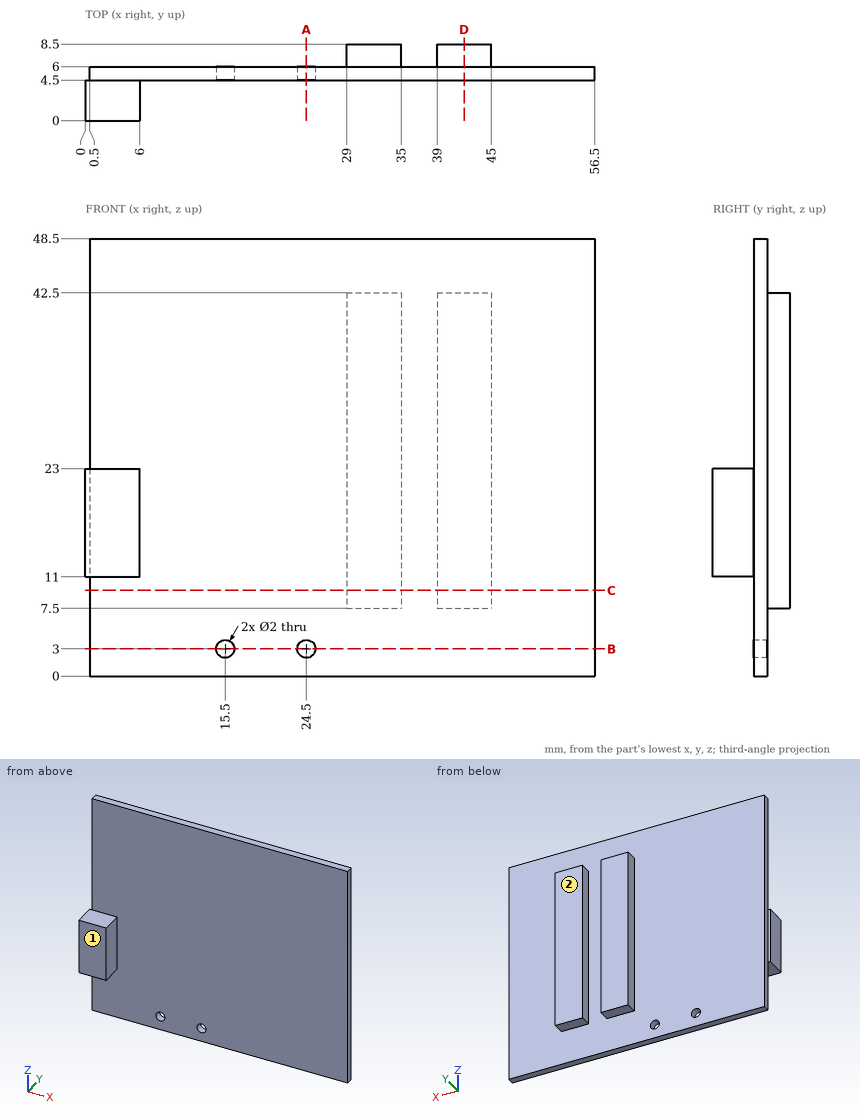
Print and shaded views of the part. All mm, measured from the part's lowest x, y and z. Coordinates: 2 decimals unless noted, no trailing zeros. Order: outer loops, then holes, each group sorted by start corner. A loop starts at its lowest first (then second) coordinate and runs counter-clockwise, first axis right, second up. Notation, with made-up numbers: M -32.75,43 L 18.25,43 A21 cw 18.25,63 Z; hole C -25,-35 d5. An arc over 180 degrees is marked long. Answer as CSV lines item,"result".
1) Mould opens along Y. For the marked faces 1 and 2 say: released by +Y, released by -Y, zero draft, split by the parting line, or undercut.
Verdict:
face 1,"released by -Y"
face 2,"released by +Y"
2) Cut at C-C (z = 9.5). List the corners of the cut face in (x, y), then the cut area to 3 significant figures.
Verdict:
outline,"M 0.5,4.5 L 56.5,4.5 L 56.5,6 L 45,6 L 45,8.5 L 39,8.5 L 39,6 L 35,6 L 35,8.5 L 29,8.5 L 29,6 L 0.5,6 Z"
area,"114 mm2"
3) Drill centre lines: L1, parallel to X at y = 5.6, z = 3; L2, parallel to X at y = 7, z = 8; L3, parallel to Y at x = 27.5, z = 9.5. Where is each one in solid material? Low to high. Write a range as from..to.
Verdict:
L1,"0.5..14.5, 16.5..23.5, 25.5..56.5"
L2,"29..35, 39..45"
L3,"4.5..6"
4) Cut at B-B (z = 3). List the corners of the cut face in (x, y).
Verdict:
outline,"M 0.5,4.5 L 14.5,4.5 L 14.5,6 L 0.5,6 Z; M 16.5,4.5 L 23.5,4.5 L 23.5,6 L 16.5,6 Z; M 25.5,4.5 L 56.5,4.5 L 56.5,6 L 25.5,6 Z"
5) Cut at D-D (x = 42). List the corners of the cut face in (y, z), then the cut area to 3 significant figures.
Verdict:
outline,"M 4.5,0 L 6,0 L 6,7.5 L 8.5,7.5 L 8.5,42.5 L 6,42.5 L 6,48.5 L 4.5,48.5 Z"
area,"160 mm2"
6) Flat gauge pins, fed straight in: P1, Ø4, axis at x = 42, y = 3, coming from the -Z side; P2, Ø1.2, axis at x = 41, y = 7, coming from the -Z side; P3, Ø1.8, axis at x = 24.5, z = 3, coming from the +Y side; P4, Ø3.5, axis at x = 4.5, y = 1.5, coming from the +Z side. Where does each tip first touch, or does it go through?
Verdict:
P1,"z = 0"
P2,"z = 7.5"
P3,"through"
P4,"z = 23"
7) Cut at A-A (x = 24.5). List the corners of the cut face in (y, z).
Verdict:
outline,"M 4.5,0 L 6,0 L 6,2 L 4.5,2 Z; M 4.5,4 L 6,4 L 6,48.5 L 4.5,48.5 Z"
